Part model, mm, in its own coordinate system. A direction names the side the tool comes from. Give positions to 0.01 mm unless a question says otherwise; leave off trailing zeros. Loops run counter-clockwise (first coordinate to the right, second up) from the corner with the lowest first, then second, coordinate; pieces in that order, holes last. Notation, with made-up numbers: M 45,7 L 73,7 A28 ccw 73,31 Z; hole C 80.5,-13.5 d6. An arc over 180 degrees is marked long. Answer in a Markdown table with one row per item.
from build123d import *

# Parameters (mm, degrees)
MAIN_BODY_DEPTH            = 12
SKETCH2_R                  = 2.55
CLEARANCE_M3_INSERTS_DEPTH = 25
CONTOURING_R               = 2


with BuildPart() as part:
    # Sketch1 → Main Body (new body, symmetric)
    with BuildSketch(Plane.XY):
        Polygon((11.25, 0), (-11.25, 0), (-11.25, 9), (-12.75, 9), (-12.75, 14), (12.75, 14), (12.75, 9), (11.25, 9), align=None)
    extrude(amount=MAIN_BODY_DEPTH, both=True)

    # Sketch2 → Clearance - M3 Inserts (cut, through all)
    with BuildSketch(Plane.ZY.offset(11.25)):
        with Locations((-7.5, 4.5)):
            Circle(SKETCH2_R)
        with Locations((7.5, 4.5)):
            Circle(SKETCH2_R)
    extrude(amount=-CLEARANCE_M3_INSERTS_DEPTH, mode=Mode.SUBTRACT)

    # Contouring
    contouring_edges = [part.edges().sort_by_distance(p)[0] for p in [
        (12, 9, -12),
        (-12, 9, 12),
        (0, 0, 12),
        (12, 9, 12),
        (0, 0, -12),
        (-12, 9, -12),
    ]]
    fillet(contouring_edges, radius=CONTOURING_R)


solid = part.part
(1) Saw through at A-A (z = 7.5). Write the cut outline in (x, y), plus the area to 3 significant figures.
Recorded:
| item | result |
|---|---|
| outline | M -12.75,9 L -11.25,9 L -11.25,7.05 L 11.25,7.05 L 11.25,9 L 12.75,9 L 12.75,14 L -12.75,14 Z; M -11.25,0 L 11.25,0 L 11.25,1.95 L -11.25,1.95 Z |
| area | 215 mm^2 |
(2) Saw through at C-C (x = 6.5). Write the cut outline in (y, z), plus the area to 3 significant figures.
Recorded:
| item | result |
|---|---|
| outline | M 0,-10 A2 ccw 2,-12 L 14,-12 L 14,12 L 2,12 A2 ccw 0,10 Z; hole C 4.5,-7.5 d5.1; hole C 4.5,7.5 d5.1 |
| area | 293 mm^2 |
(3) Saw through at D-D (z = -3). Write the cut outline in (x, y).
Recorded:
| item | result |
|---|---|
| outline | M -12.75,9 L -11.25,9 L -11.25,0 L 11.25,0 L 11.25,9 L 12.75,9 L 12.75,14 L -12.75,14 Z |
(4) Pin check, flat tips, straight feed: pin 1 Ø0.8 at (x, z) = (12, 1) entering from -Y; pin 2 Ø4.5 at (y, z) = (4.5, 7.5) entering from -X; pin 3 Ø3 at (y, z) = (6, 9.5) entering from -X; pin 4 Ø5.5 at (y, z) = (6.5, 5) entering from -X. Stop position of each tip, or through.
Recorded:
| item | result |
|---|---|
| pin 1 | stops at y = 9 |
| pin 2 | passes through |
| pin 3 | stops at x = -11.25 |
| pin 4 | stops at x = -12.75 |
(5) Pull direction Y, two halves, no side cores. Call faces 4 (the face through (11.99, 9.6, -11.43)), 5 (the face through (11.25, 4, 0)), 6 (the face through (-0.16, 6.65, -6.13)): +Y half, -Y half, draft (parallel to the pull), parting line (faces both ways), or undercut.
Recorded:
| item | result |
|---|---|
| face 4 | -Y half |
| face 5 | draft |
| face 6 | undercut |
(6) Which spindle directions (+Z, -Z, +X, -X, +Y, -Y) get a long thin tool onto all of the face, cutting with end or side? Do faces 1 (the face through (-12, 9, 0)), 2 (the face through (-12.01, 9.6, -11.43)), 3 (the face through (11.99, 9.6, 11.43)). Say none if no direction does.
Recorded:
| item | result |
|---|---|
| face 1 | +Z, -Z, -X, -Y |
| face 2 | -Z, -X, -Y |
| face 3 | +Z, +X, -Y |
(7) Drill centre lines: line 1 along Y through (x, z) = (-1.25, -7.5); line 2 along Z through (x, y) = (-6.25, 3); line 3 along X through (y, z) = (8.5, -3.5). Where is each one in solid material? Low to high.
Recorded:
| item | result |
|---|---|
| line 1 | y = 0 to 1.95, 7.05 to 14 |
| line 2 | z = -12 to -9.56, -5.44 to 5.44, 9.56 to 12 |
| line 3 | x = -11.25 to 11.25 |
(8) Saw through at B-B (y = 4.5). Write the cut outline in (x, z).
Recorded:
| item | result |
|---|---|
| outline | M -11.25,-12 L 11.25,-12 L 11.25,-10.05 L -11.25,-10.05 Z; M -11.25,-4.95 L 11.25,-4.95 L 11.25,4.95 L -11.25,4.95 Z; M -11.25,10.05 L 11.25,10.05 L 11.25,12 L -11.25,12 Z |
